Could you check a few things on this model? Use its own coordinates, in mm. Give positions to 0.01 mm unless a question says otherwise; leave off trailing zeros. Order: outer loops, then holes, each group sorted by start corner. A loop starts at its lowest first (then second) coordinate and runs counter-clockwise, first axis right, second up. Notation, with made-up numbers: (62, 64) - (66, 64) arc R5 cw to (66, 71) - close; hole circle Ø5 at (64, -17). An arc over 180 degrees is marked (long way). Put each result on its own line as item: value.
Autodesk Inventor part; units mm, degrees
ref_plane "YZ Plane" through (0, 0, 0) normal (1, 0, 0) x (0, 1, 0)
ref_plane "XZ Plane" through (0, 0, 0) normal (0, 1, 0) x (-1, 0, 0)
ref_plane "XY Plane" through (0, 0, 0) normal (0, 0, 1) x (1, 0, 0)
sketch "Эскиз2" plane through (0, 0, 0) normal (0, 0, 1) x (1, 0, 0)
  line L0 (80, 60) -> (0, 60)
  line L1 (0, 60) -> (0, -60)
  line L2 (0, -60) -> (80, -60)
  line L3 (80, -60) -> (80, 60)
  line L4 (80, 60) -> (78, 60)
  line L5 (78, 60) -> (78, 58)
  line L6 (78, 58) -> (80, 58)
  line L7 (80, 58) -> (80, 60)
  circle A0 centre (78, 58) radius 1.5
  line L8 (80, 0) -> (0, 0) construction
  circle A1 centre (78, -58) radius 1.5
  line L9 (40, 0) -> (40, 60) construction
  circle A2 centre (2, 58) radius 1.5
  circle A3 centre (2, -58) radius 1.5
  point P0 (79.5, 58)
  point P1 (78, 59.5)
  dimension "d5" = 120
  dimension "d6" = 2
  dimension "d7" = 2
  dimension "d8" = 3
sketch "Эскиз3" plane through (0, 0, 0) normal (0, 0, 1) x (1, 0, 0)
  circle A0 centre (78, 57.9993) radius 1.5
  line L0 (79.5, 0) -> (0, 0)
  line L1 (0, 0) -> (40, 0) construction
  line L2 (40, 0) -> (40, 1.7902)
  line L3 (40, 1.7902) -> (40, 59.4993) construction
  circle A1 centre (78, -57.9993) radius 1.5
  circle A2 centre (2, 57.9993) radius 1.5
  circle A3 centre (2, -57.9993) radius 1.5
  dimension "d11" = 3
  dimension "d12" = 40
extrude "Выдавливание1" add sketch "Эскиз3" along normal blind 5
extrude "Выдавливание2" add sketch "Эскиз2" along normal blind 1 from surface at 5 contours L5 A0 L6 L3 L2 L1 L0
sketch "Эскиз4" plane through (0, -60, 6) normal (0, 0, 1) x (1, 0, 0)
  point P0 (0, 60)
sketch "Эскиз5" plane through (0, -60, 6) normal (0, 0, 1) x (1, 0, 0)
  circle A0 centre (78, 117.9993) radius 1.5
  line L0 (78, 117.9993) -> (89, 117.9993) construction
  circle A1 centre (64.4943, 115.9487) radius 1.5
  circle A2 centre (75.9494, 104.4935) radius 1.5
  line L1 (80, 118) -> (80, 0)
  circle A3 centre (64.4943, 4.0513) radius 1.5
  circle A4 centre (75.9494, 15.5065) radius 1.5
  point P0 (0, 60)
  dimension "d21" = 3
  dimension "d22" = 3
extrude "Выдавливание3" cut sketch "Эскиз5" against normal blind 1 contours A1 | A2 | A3 | A4
properties part number "макетная плата"
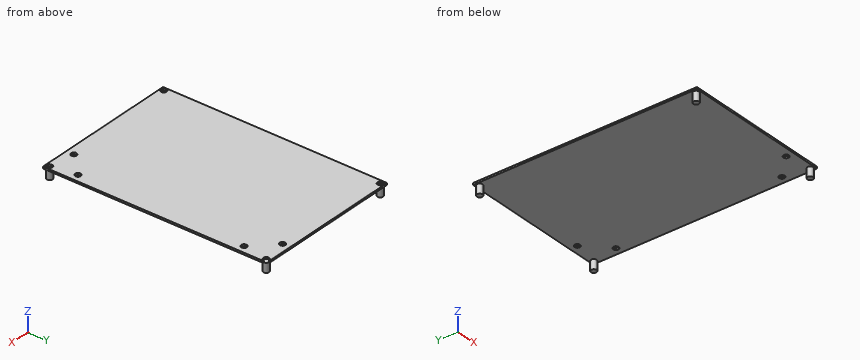
1) Suppose I cut it at D-D, the plane x = 23. List the corners of the cut face in (y, z) for me.
Filled in:
outline: (-60, 5) - (60, 5) - (60, 6) - (-60, 6) - close
2) Suppose I cut it at B-B, the plane y = 41. List the corners of the cut face in (x, z) for me, and give its area (3 significant figures).
Filled in:
outline: (0, 5) - (80, 5) - (80, 6) - (0, 6) - close
area: 80.0 mm^2
3) Suppose I cut it at A-A, the plane x = 2. List the corners of the cut face in (y, z) for me.
Filled in:
outline: (-60, 5) - (-59.5, 5) - (-59.5, 6) - (-60, 6) - close; (-59.5, 0) - (-56.5, 0) - (-56.5, 5) - (56.5, 5) - (56.5, 0) - (59.5, 0) - (59.5, 5) - (56.5, 5) - (56.5, 6) - (-56.5, 6) - (-56.5, 5) - (-59.5, 5) - close; (59.5, 5) - (60, 5) - (60, 6) - (59.5, 6) - close
4) If I drill on line 1 (Y direction, x = 2, z = 5.7); line 2 (Z direction, x = 25, y = -31.5), over which ranges is the centre line in solid material (lowest first)? Write a range as [from, to].
Filled in:
line 1: y = [-60, -59.5], [-56.5, 56.5], [59.5, 60]
line 2: z = [5, 6]
5) I'm going to push flat-ended pins straight in: pin 1 (4 mm diameter, centred on x = 64.49, y = 55.95, fed in from -Z); pin 2 (2.5 mm diameter, centred on x = 78, y = 58, fed in from +Z); pin 3 (0.6 mm diameter, centred on y = 59.5, z = 5.5, fed in from +X). Where does each tip first touch, or does it pass through?
Filled in:
pin 1: stops at z = 5
pin 2: stops at z = 5
pin 3: stops at x = 78
6) Suppose I cut it at C-C, the plane z = 2.45. List the corners of the cut face in (x, y) for me, and give its area (3 significant figures).
Filled in:
outline: circle Ø3 at (2, -58); circle Ø3 at (2, 58); circle Ø3 at (78, -58); circle Ø3 at (78, 58)
area: 28.3 mm^2
